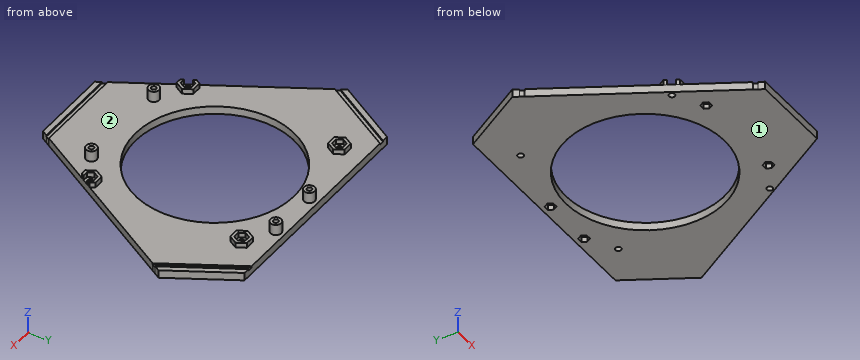
```python
from build123d import *

# Parameters (mm, degrees)
F2_DEPTH      = 5.5
F3_DEPTH      = 4.5
F4_R          = 3.7
F4_R_2        = 1.7
F5_DEPTH      = 7.5
F6_DEPTH      = 25
F7_R          = 2
F7_R_2        = 55
F8_DEPTH      = 25
F9_DEPTH      = 7.5
F9_DEPTH_BACK = 2
F10_START     = -1.6
F10_DEPTH     = 0.4
F12_DEPTH     = 3.5
F14_W         = 250.9568184614
F14_H         = 134.5421932638
F15_DEPTH     = 25


with BuildPart() as f2:
    # F1 (on face) → F2 (new body)
    with BuildSketch(Plane.XY):
        Polygon((-66.2961039686, 74.7239265275), (-97.8608706276, 20.052146945), (-31.5647666591, -94.7760734725), (31.5647666591, -94.7760734725), (97.8608706276, 20.052146945), (66.2961039686, 74.7239265275), align=None)
    extrude(amount=F2_DEPTH)



with BuildPart() as f2b:
    # F1 (on face) → F2, piece 2 (new body)
    with BuildSketch(Plane.XY):
        Polygon((73.801657468, 74.7239265275), (69.529265476, 74.7239265275), (99.4774513814, 22.852146945), (101.6136473774, 26.552146945), align=None)
    extrude(amount=F2_DEPTH)


with BuildPart() as f2c:
    # F1 (on face) → F2, piece 3 (new body)
    with BuildSketch(Plane.XY):
        Polygon((29.9481859053, -97.5760734725), (-29.9481859053, -97.5760734725), (-27.8119899093, -101.2760734725), (27.8119899093, -101.2760734725), align=None)
    extrude(amount=F2_DEPTH)


with BuildPart() as f2d:
    # F1 (on face) → F2, piece 4 (new body)
    with BuildSketch(Plane.XY):
        Polygon((-73.801657468, 74.7239265275), (-101.6136473774, 26.552146945), (-99.4774513814, 22.852146945), (-69.529265476, 74.7239265275), align=None)
    extrude(amount=F2_DEPTH)


with BuildPart() as f2_1:
    add(f2.part)

    add(f2b.part)  # F3 merges F2b

    add(f2c.part)  # F3 merges F2c

    add(f2d.part)  # F3 merges F2d
    # F1 (on face) → F3 (join)
    with BuildSketch(Plane.XY):
        Polygon((-69.529265476, 74.7239265275), (-99.4774513814, 22.852146945), (-98.1495457622, 20.552146945), (-66.8734542378, 74.7239265275), align=None)
        Polygon((31.2760915245, -95.2760734725), (-31.2760915245, -95.2760734725), (-29.9481859053, -97.5760734725), (29.9481859053, -97.5760734725), align=None)
        Polygon((31.5647666591, -94.7760734725), (-31.5647666591, -94.7760734725), (-31.2760915245, -95.2760734725), (31.2760915245, -95.2760734725), align=None)
        Polygon((66.8734542378, 74.7239265275), (66.2961039686, 74.7239265275), (97.8608706276, 20.052146945), (98.1495457622, 20.552146945), align=None)
        Polygon((69.529265476, 74.7239265275), (66.8734542378, 74.7239265275), (98.1495457622, 20.552146945), (99.4774513814, 22.852146945), align=None)
        Polygon((-66.8734542378, 74.7239265275), (-98.1495457622, 20.552146945), (-97.8608706276, 20.052146945), (-66.2961039686, 74.7239265275), align=None)
    extrude(amount=F3_DEPTH)

    # F4 (on face) → F5 (join)
    with BuildSketch(Plane.XY.offset(5.5)):
        with Locations((33.5, 64)):
            Circle(F4_R)
        with Locations((33.5, 64)):
            Circle(F4_R_2, mode=Mode.SUBTRACT)
        with Locations((-2.5, 64)):
            Circle(F4_R)
        with Locations((-2.5, 64)):
            Circle(F4_R_2, mode=Mode.SUBTRACT)
        with Locations((33.5, -64)):
            Circle(F4_R)
        with Locations((33.5, -64)):
            Circle(F4_R_2, mode=Mode.SUBTRACT)
        with Locations((-33.5, -64)):
            Circle(F4_R)
        with Locations((-33.5, -64)):
            Circle(F4_R_2, mode=Mode.SUBTRACT)
    extrude(amount=F5_DEPTH)

    # F6 (cut): faces of the model
    f6_faces = [f2_1.faces().sort_by_distance(p)[0] for p in [
        (-33.5, -64, 5.5),
        (33.5, -64, 5.5),
        (-2.5, 64, 5.5),
        (33.5, 64, 5.5),
    ]]
    extrude(f6_faces, amount=-F6_DEPTH, mode=Mode.SUBTRACT)

    # F7 (on face) → F8 (cut)
    with BuildSketch(Plane.XY):
        with Locations((52.5, 52.5)):
            Circle(F7_R)
        with Locations((52.5, -52.5)):
            Circle(F7_R)
        with Locations((-52.5, -52.5)):
            Circle(F7_R)
        with Locations((-52.5, 52.5)):
            Circle(F7_R)
        Circle(F7_R_2)
        Polygon((-31.7679491924, -67), (-30.0358983849, -64), (-31.7679491924, -61), (-35.2320508076, -61), (-36.9641016151, -64), (-35.2320508076, -67), align=None)
        Polygon((31.7679491924, -67), (35.2320508076, -67), (36.9641016151, -64), (35.2320508076, -61), (31.7679491924, -61), (30.0358983849, -64), align=None)
        Polygon((-4.2320508076, 61), (-0.7679491924, 61), (0.9641016151, 64), (-0.7679491924, 67), (-4.2320508076, 67), (-5.9641016151, 64), align=None)
        Polygon((31.7679491924, 61), (35.2320508076, 61), (36.9641016151, 64), (35.2320508076, 67), (31.7679491924, 67), (30.0358983849, 64), align=None)
    extrude(amount=F8_DEPTH, mode=Mode.SUBTRACT)

    # F4 (on face) → F9 (join, two sides)
    with BuildSketch(Plane.XY.offset(5.5)) as f9_sk:
        with Locations((33.5, 64)):
            Circle(F4_R)
        with Locations((33.5, 64)):
            Circle(F4_R_2, mode=Mode.SUBTRACT)
        with Locations((-2.5, 64)):
            Circle(F4_R)
        with Locations((-2.5, 64)):
            Circle(F4_R_2, mode=Mode.SUBTRACT)
        with Locations((33.5, -64)):
            Circle(F4_R)
        with Locations((33.5, -64)):
            Circle(F4_R_2, mode=Mode.SUBTRACT)
        with Locations((-33.5, -64)):
            Circle(F4_R)
        with Locations((-33.5, -64)):
            Circle(F4_R_2, mode=Mode.SUBTRACT)
    extrude(amount=F9_DEPTH)
    extrude(f9_sk.sketch, amount=-F9_DEPTH_BACK)

    # F4 (on face) → F10 (join)
    with BuildSketch(Plane.XY.offset(5.5).offset(F10_START)):
        with Locations((33.5, 64)):
            Circle(F4_R_2)
        with Locations((-2.5, 64)):
            Circle(F4_R_2)
        with Locations((-33.5, -64)):
            Circle(F4_R_2)
        with Locations((33.5, -64)):
            Circle(F4_R_2)
    extrude(amount=-F10_DEPTH)

    # F11 (on face) → F12 (join)
    with BuildSketch(Plane.XY.offset(5.5)):
        Polygon((-56.4014980388, -51.7575928288), (-54.6650635095, -48.75), (-50.3349364905, -48.75), (-48.1698729811, -52.5), (-50.3349364905, -56.25), (-53.8078055492, -56.25), (-52.6531050108, -58.25), (-49.1802359522, -58.25), (-45.8604719043, -52.5), (-49.1802359522, -46.75), (-55.8197640478, -46.75), (-57.5561985772, -49.7575928288), align=None)
        Polygon((49.1802359522, -58.25), (52.6531050108, -58.25), (53.8078055492, -56.25), (50.3349364905, -56.25), (48.1698729811, -52.5), (50.3349364905, -48.75), (54.6650635095, -48.75), (56.4014980388, -51.7575928288), (57.5561985772, -49.7575928288), (55.8197640478, -46.75), (49.1802359522, -46.75), (45.8604719043, -52.5), align=None)
        Polygon((-55.8197640478, 46.75), (-49.1802359522, 46.75), (-45.8604719043, 52.5), (-49.1802359522, 58.25), (-55.8197640478, 58.25), (-59.1395280957, 52.5), align=None)
        Polygon((-48.1698729811, 52.5), (-50.3349364905, 48.75), (-54.6650635095, 48.75), (-56.8301270189, 52.5), (-54.6650635095, 56.25), (-50.3349364905, 56.25), align=None, mode=Mode.SUBTRACT)
        Polygon((49.1802359522, 46.75), (55.8197640478, 46.75), (59.1395280957, 52.5), (55.8197640478, 58.25), (49.1802359522, 58.25), (45.8604719043, 52.5), align=None)
        Polygon((56.8301270189, 52.5), (54.6650635095, 48.75), (50.3349364905, 48.75), (48.1698729811, 52.5), (50.3349364905, 56.25), (54.6650635095, 56.25), align=None, mode=Mode.SUBTRACT)
    extrude(amount=F12_DEPTH)

    # F14 (on offset) → F15 (cut)
    with BuildSketch(Plane.XZ.offset(-70)):
        with Locations((4.6517625451, 26.0684285313)):
            Rectangle(F14_W, F14_H)
    extrude(amount=-F15_DEPTH, mode=Mode.SUBTRACT)


solid = f2_1.part
```
Check sheet for the modelled part. Datum: model origin and axes. Units: mm. Face numbers are marked on the shaded views. Give positions to 0.01 mm unless a question says otherwise; leave off trailing zeros. Write each loop counter-clockwise with the first axis right and the second up, starting at its lowest first coordinate (ties: lowest second). Pieces come first, ordered by that corner, then holes.
Item 1: Cross-section at D-D (x = 5.5). Enter the section's corners in (y, z), and give its area (3 significant figures).
Item 2: Cross-section at B-B (y = -38). Enter the section's corners in (x, z), and give its area (3 significant figures).
Item 3: Cross-section at A-A (x = -15). Enter the section's corners in (y, z), and give its area (3 significant figures).
Item 4: Draft check along X on the marked faces 1 and 2. Enter one of: released by +X, released by -X, zero draft, split by the parting line, or undercut.
Item 5: Scan lines: L1, parallel to X at y = 64, z = 5; L2, parallel to Y at x = 33.5, z = 4.85; L3, parallel to Y at x = -2.5, z = 8.25. Record each from-to range of solid material in increasing order.
Item 6: Gauge pin test, flat ends, axial feed: pin 1 (12 mm diameter, centred on x = 37, y = -23, fed in from +Z); pin 2 (1.5 mm diameter, centred on y = -66, z = 6.5, fed in from +X); pin 3 (1 mm diameter, centred on y = 30, z = 5, fed in from +X); pin 4 (6 mm diameter, centred on y = -13.5, z = 7.5, fed in from +X). Record the tip position at first contact, or that the pin passes through.
Item 7: Cross-section at C-C (y = 15.5). Enter the section's corners in (x, z), and give its area (3 significant figures).
Report:
1. outline: (-101.28, 0) - (-54.72, 0) - (-54.72, 5.5) - (-94.78, 5.5) - (-94.78, 4.5) - (-97.58, 4.5) - (-97.58, 5.5) - (-101.28, 5.5) - close; (54.72, 0) - (70, 0) - (70, 5.5) - (54.72, 5.5) - close
1. area: 337 mm2
2. outline: (-64.34, 0) - (-39.76, 0) - (-39.76, 5.5) - (-64.34, 5.5) - close; (39.76, 0) - (64.34, 0) - (64.34, 5.5) - (39.76, 5.5) - close
2. area: 270 mm2
3. outline: (-101.28, 0) - (-52.92, 0) - (-52.92, 5.5) - (-94.78, 5.5) - (-94.78, 4.5) - (-97.58, 4.5) - (-97.58, 5.5) - (-101.28, 5.5) - close; (52.92, 0) - (70, 0) - (70, 5.5) - (52.92, 5.5) - close
3. area: 357 mm2
4. face 1: zero draft
4. face 2: undercut
5. L1: x = -79.99 to -75.72, -72.49 to -4.2, -0.8 to 31.8, 35.2 to 72.49, 75.72 to 79.99
5. L2: y = -91.42 to -65.7, -62.3 to -43.62, 43.62 to 62.3, 65.7 to 70
5. L3: y = 60.3 to 62.3, 65.7 to 67.7
6. pin 1: passes through
6. pin 2: stops at x = 36.98
6. pin 3: stops at x = 99.91
6. pin 4: stops at x = 79.78
7. outline: (-95.23, 0) - (-52.77, 0) - (-52.77, 5.5) - (-95.23, 5.5) - close; (52.77, 0) - (95.23, 0) - (95.23, 5.5) - (52.77, 5.5) - close
7. area: 467 mm2
